Check sheet for the modelled part. Datum: model origin and axes. Units: mm. Round coordinates to 2 decimals unless told otherwise and drop trailing zeros. Loops run counter-clockwise (first coordinate to the right, second up) from the corner with the lowest first, then second, coordinate; pieces in that order, holes last. Notation, with made-up numbers: (-15.5, 51) -> (15.5, 51) arc R18 ccw to (15.5, 77) -> close; hole circle Ø11 at (36.25, 64.25). An arc over 180 degrees is marked (long way). One line per question, with ' | ' between items.
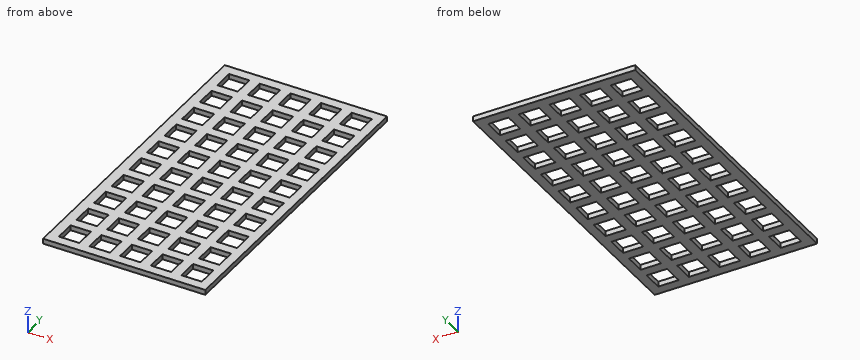
```python
from build123d import *

# Parameters (mm, degrees)
SKETCH1_W           = 79.5
SKETCH1_H           = 154.8
SKETCH1_W_2         = 10
SKETCH1_H_2         = 10
BOSS_EXTRUDE1_DEPTH = 2.5


with BuildPart() as part:
    # Sketch1 → Boss-Extrude1 (new body)
    with BuildSketch(Plane.XY):
        with Locations((39.75, -77.4)):
            Rectangle(SKETCH1_W, SKETCH1_H)
        with Locations((10, -10)):
            Rectangle(SKETCH1_W_2, SKETCH1_H_2, mode=Mode.SUBTRACT)
        with Locations((25, -10)):
            Rectangle(SKETCH1_W_2, SKETCH1_H_2, mode=Mode.SUBTRACT)
        with Locations((40, -10)):
            Rectangle(SKETCH1_W_2, SKETCH1_H_2, mode=Mode.SUBTRACT)
        with Locations((55, -10)):
            Rectangle(SKETCH1_W_2, SKETCH1_H_2, mode=Mode.SUBTRACT)
        with Locations((70, -10)):
            Rectangle(SKETCH1_W_2, SKETCH1_H_2, mode=Mode.SUBTRACT)
        with Locations((25, -25)):
            Rectangle(SKETCH1_W_2, SKETCH1_H_2, mode=Mode.SUBTRACT)
        with Locations((40, -25)):
            Rectangle(SKETCH1_W_2, SKETCH1_H_2, mode=Mode.SUBTRACT)
        with Locations((55, -25)):
            Rectangle(SKETCH1_W_2, SKETCH1_H_2, mode=Mode.SUBTRACT)
        with Locations((70, -25)):
            Rectangle(SKETCH1_W_2, SKETCH1_H_2, mode=Mode.SUBTRACT)
        with Locations((25, -40)):
            Rectangle(SKETCH1_W_2, SKETCH1_H_2, mode=Mode.SUBTRACT)
        with Locations((40, -40)):
            Rectangle(SKETCH1_W_2, SKETCH1_H_2, mode=Mode.SUBTRACT)
        with Locations((55, -40)):
            Rectangle(SKETCH1_W_2, SKETCH1_H_2, mode=Mode.SUBTRACT)
        with Locations((70, -40)):
            Rectangle(SKETCH1_W_2, SKETCH1_H_2, mode=Mode.SUBTRACT)
        with Locations((25, -55)):
            Rectangle(SKETCH1_W_2, SKETCH1_H_2, mode=Mode.SUBTRACT)
        with Locations((40, -55)):
            Rectangle(SKETCH1_W_2, SKETCH1_H_2, mode=Mode.SUBTRACT)
        with Locations((55, -55)):
            Rectangle(SKETCH1_W_2, SKETCH1_H_2, mode=Mode.SUBTRACT)
        with Locations((70, -55)):
            Rectangle(SKETCH1_W_2, SKETCH1_H_2, mode=Mode.SUBTRACT)
        with Locations((25, -70)):
            Rectangle(SKETCH1_W_2, SKETCH1_H_2, mode=Mode.SUBTRACT)
        with Locations((40, -70)):
            Rectangle(SKETCH1_W_2, SKETCH1_H_2, mode=Mode.SUBTRACT)
        with Locations((55, -70)):
            Rectangle(SKETCH1_W_2, SKETCH1_H_2, mode=Mode.SUBTRACT)
        with Locations((70, -70)):
            Rectangle(SKETCH1_W_2, SKETCH1_H_2, mode=Mode.SUBTRACT)
        with Locations((25, -85)):
            Rectangle(SKETCH1_W_2, SKETCH1_H_2, mode=Mode.SUBTRACT)
        with Locations((40, -85)):
            Rectangle(SKETCH1_W_2, SKETCH1_H_2, mode=Mode.SUBTRACT)
        with Locations((55, -85)):
            Rectangle(SKETCH1_W_2, SKETCH1_H_2, mode=Mode.SUBTRACT)
        with Locations((70, -85)):
            Rectangle(SKETCH1_W_2, SKETCH1_H_2, mode=Mode.SUBTRACT)
        with Locations((25, -100)):
            Rectangle(SKETCH1_W_2, SKETCH1_H_2, mode=Mode.SUBTRACT)
        with Locations((40, -100)):
            Rectangle(SKETCH1_W_2, SKETCH1_H_2, mode=Mode.SUBTRACT)
        with Locations((55, -100)):
            Rectangle(SKETCH1_W_2, SKETCH1_H_2, mode=Mode.SUBTRACT)
        with Locations((70, -100)):
            Rectangle(SKETCH1_W_2, SKETCH1_H_2, mode=Mode.SUBTRACT)
        with Locations((25, -115)):
            Rectangle(SKETCH1_W_2, SKETCH1_H_2, mode=Mode.SUBTRACT)
        with Locations((40, -115)):
            Rectangle(SKETCH1_W_2, SKETCH1_H_2, mode=Mode.SUBTRACT)
        with Locations((55, -115)):
            Rectangle(SKETCH1_W_2, SKETCH1_H_2, mode=Mode.SUBTRACT)
        with Locations((70, -115)):
            Rectangle(SKETCH1_W_2, SKETCH1_H_2, mode=Mode.SUBTRACT)
        with Locations((25, -130)):
            Rectangle(SKETCH1_W_2, SKETCH1_H_2, mode=Mode.SUBTRACT)
        with Locations((40, -130)):
            Rectangle(SKETCH1_W_2, SKETCH1_H_2, mode=Mode.SUBTRACT)
        with Locations((55, -130)):
            Rectangle(SKETCH1_W_2, SKETCH1_H_2, mode=Mode.SUBTRACT)
        with Locations((70, -130)):
            Rectangle(SKETCH1_W_2, SKETCH1_H_2, mode=Mode.SUBTRACT)
        with Locations((25, -145)):
            Rectangle(SKETCH1_W_2, SKETCH1_H_2, mode=Mode.SUBTRACT)
        with Locations((40, -145)):
            Rectangle(SKETCH1_W_2, SKETCH1_H_2, mode=Mode.SUBTRACT)
        with Locations((55, -145)):
            Rectangle(SKETCH1_W_2, SKETCH1_H_2, mode=Mode.SUBTRACT)
        with Locations((70, -145)):
            Rectangle(SKETCH1_W_2, SKETCH1_H_2, mode=Mode.SUBTRACT)
        with Locations((10, -25)):
            Rectangle(SKETCH1_W_2, SKETCH1_H_2, mode=Mode.SUBTRACT)
        with Locations((10, -40)):
            Rectangle(SKETCH1_W_2, SKETCH1_H_2, mode=Mode.SUBTRACT)
        with Locations((10, -55)):
            Rectangle(SKETCH1_W_2, SKETCH1_H_2, mode=Mode.SUBTRACT)
        with Locations((10, -70)):
            Rectangle(SKETCH1_W_2, SKETCH1_H_2, mode=Mode.SUBTRACT)
        with Locations((10, -85)):
            Rectangle(SKETCH1_W_2, SKETCH1_H_2, mode=Mode.SUBTRACT)
        with Locations((10, -100)):
            Rectangle(SKETCH1_W_2, SKETCH1_H_2, mode=Mode.SUBTRACT)
        with Locations((10, -115)):
            Rectangle(SKETCH1_W_2, SKETCH1_H_2, mode=Mode.SUBTRACT)
        with Locations((10, -130)):
            Rectangle(SKETCH1_W_2, SKETCH1_H_2, mode=Mode.SUBTRACT)
        with Locations((10, -145)):
            Rectangle(SKETCH1_W_2, SKETCH1_H_2, mode=Mode.SUBTRACT)
    extrude(amount=BOSS_EXTRUDE1_DEPTH)


solid = part.part
```
(1) Go/stop test with flat-tipped pins: pin 1 (6 mm diameter, centred on x = 37, y = -129.5, fed in from -Z); pin 2 (3 mm diameter, centred on x = 13, y = -69.5, fed in from -Z). Record where each tip stops, or that it passes through.
Answer:
pin 1: stops at z = 0 | pin 2: passes through
(2) Sectioned sample at A-A, the plane y = -55.5. Record the cut outline in (x, z).
Answer:
outline: (0, 0) -> (5, 0) -> (5, 2.5) -> (0, 2.5) -> close; (15, 0) -> (20, 0) -> (20, 2.5) -> (15, 2.5) -> close; (30, 0) -> (35, 0) -> (35, 2.5) -> (30, 2.5) -> close; (45, 0) -> (50, 0) -> (50, 2.5) -> (45, 2.5) -> close; (60, 0) -> (65, 0) -> (65, 2.5) -> (60, 2.5) -> close; (75, 0) -> (79.5, 0) -> (79.5, 2.5) -> (75, 2.5) -> close
(3) Scan line: probe 1 along X at (y, z) = (-147.5, 0.4). Record every from-to range of solid material in increasing order.
Answer:
probe 1: x = 0 to 5, 15 to 20, 30 to 35, 45 to 50, 60 to 65, 75 to 79.5
(4) Sectioned sample at B-B, the plane z = 1.7. Count the separate pieces of the cut face and the enclosed holes in it, and give its area (3 significant figures).
Answer:
separate pieces: 1 | enclosed holes: 50 | area: 7,310 mm2
